from build123d import *

# Parameters (mm, degrees)
SKETCH1_R           = 1.5
BOSS_EXTRUDE1_DEPTH = 1.1
SKETCH2_R           = 2.455
BOSS_EXTRUDE2_DEPTH = 7.365
DOME1_FACE_RADIUS   = 2.455
DOME1_HEIGHT        = 2.455
SKETCH9_W           = 6
SKETCH9_H           = 9.85
BOSS_EXTRUDE3_DEPTH = 5.52
BOSS_EXTRUDE4_DEPTH = 9.85


with BuildPart() as part:
    # Sketch1 → Boss-Extrude1 (new body)
    with BuildSketch(Plane(origin=(0, 0, 0), x_dir=(1, 0, 0), z_dir=(0, 1, 0))):
        with BuildLine():
            Line((3.5, 0), (26.5, 0))
            ThreePointArc((26.5, 0), (28.974873734, 1.025126266), (30, 3.5))
            Line((30, 3.5), (30, 18.5))
            ThreePointArc((30, 18.5), (28.974873734, 20.974873734), (26.5, 22))
            Line((26.5, 22), (3.5, 22))
            ThreePointArc((3.5, 22), (1.025126266, 20.974873734), (0, 18.5))
            Line((0, 18.5), (0, 3.5))
            ThreePointArc((0, 3.5), (1.025126266, 1.025126266), (3.5, 0))
        make_face()
        with Locations(Location((26.5, 18.5, 0), (0, 0, 270))):
            Circle(SKETCH1_R, mode=Mode.SUBTRACT)
        with Locations(Location((26.5, 3.5, 0), (0, 0, 270))):
            Circle(SKETCH1_R, mode=Mode.SUBTRACT)
    extrude(amount=BOSS_EXTRUDE1_DEPTH)

    # Sketch2 → Boss-Extrude2 (add)
    with BuildSketch(Plane(origin=(0, 1.1, 0), x_dir=(1, 0, 0), z_dir=(0, 1, 0))):
        with Locations(Location((17.375, 11, 0), (0, 0, 270))):
            Circle(SKETCH2_R)
    extrude(amount=BOSS_EXTRUDE2_DEPTH)

    # Dome1: a dome of height H over a round flat face of radius A is a cap of a sphere of radius (A * A + H * H) / (2 * H)
    dome1_r = (DOME1_FACE_RADIUS * DOME1_FACE_RADIUS + DOME1_HEIGHT * DOME1_HEIGHT) / (2 * DOME1_HEIGHT)
    dome1_base = Plane((17.375, 8.465, -11), z_dir=(0, 1, 0))
    with Locations(dome1_base.offset(DOME1_HEIGHT - dome1_r)):
        dome1_ball = Sphere(dome1_r, mode=Mode.PRIVATE)
    add(split(dome1_ball, bisect_by=dome1_base, keep=Keep.TOP, mode=Mode.PRIVATE))

    # Sketch9 → Boss-Extrude3 (add)
    with BuildSketch(Plane(origin=(0, 1.1, 0), x_dir=(1, 0, 0), z_dir=(0, 1, 0))):
        with Locations((3, 11)):
            Rectangle(SKETCH9_W, SKETCH9_H)
    extrude(amount=BOSS_EXTRUDE3_DEPTH)

    # Sketch11 → Boss-Extrude4 (add)
    with BuildSketch(Plane(origin=(0, 0, -15.925), x_dir=(-1, 0, 0), z_dir=(0, 0, -1))):
        Polygon((0, 1.1), (-7.61, 1.1), (-6, 6.62), (0, 6.62), align=None)
    extrude(amount=-BOSS_EXTRUDE4_DEPTH)


solid = part.part
The listing builds one solid part. Answer for the finished solid, in the listing's coordinates (mm). A direction names the side the tool comes from. Give positions to 0.01 mm unless a question says otherwise; leave off trailing zeros. Loops run counter-clockwise (first coordinate to the right, second up) from the corner with the lowest first, then second, coordinate; pieces in that order, holes last. Notation, with made-up numbers: (85, -6) - (113, -6) arc R20 cw to (113, 18) - close; hole circle Ø10 at (23.5, 42.25). An arc over 180 degrees is marked (long way). Answer as a JSON object with one key per item and string values.
1. A cutting plane is placed at A-A (z = -11). Write down the section's boundary in (x, y) (3 decimals).
Determined:
{"outline": "(0, 0) - (30, 0) - (30, 1.1) - (19.83, 1.1) - (19.83, 8.465) arc R2.455 ccw to (14.92, 8.465) - (14.92, 1.1) - (7.61, 1.1) - (6, 6.62) - (0, 6.62) - close"}
2. Flat-ended cylindrical pins translate along their axes: pin 1 Ø1.7 at (x, y) = (3.5, 5) entering from -Z (3 decimals); pin 2 Ø1.7 at (x, y) = (3.5, 3) entering from +Z (3 decimals); pin 3 Ø6.5 at (x, z) = (2, -10.5) entering from +Y. Find the tip coordinate at first contact, or state that the pin passes through.
Determined:
{"pin 1": "z = -15.925", "pin 2": "z = -6.075", "pin 3": "y = 6.62"}
3. A cutting plane is placed at D-D (x = 9.5). Write down the section's boundary in (y, z), then the cut area to 3 significant figures.
Determined:
{"outline": "(0, -22) - (1.1, -22) - (1.1, 0) - (0, 0) - close", "area": "24.2 mm²"}
4. For a pull along X with two mould halves and no side action, classify faces 5 (the cylindrical face through (29, 0.54, -20.95)), 6 (the cylindrical face through (27.765, 0.542, -2.694)), 7 (the cylindrical face through (1, 0.54, -1.05)), 8 (the flat face through (4, 4, -15.925)) as pulls with the +X half, pulls with the -X half, needs draft (parallel to the pull), parting line crosses it, or undercut.
Determined:
{"face 5": "pulls with the +X half", "face 6": "undercut", "face 7": "pulls with the -X half", "face 8": "needs draft"}
5. A cutting plane is placed at C-C (y = 8). Write down the section's boundary in (x, z) (3 decimals).
Determined:
{"outline": "circle Ø4.91 at (17.375, -11)"}
6. Find the intervals of material crossed by L1, parallel to X at y = 0.75, z = -18.5; L2, parallel to Y at x = 8.5, z = -13; L3, parallel to Z at x = 6.75, y = 2 (3 decimals), in increasing order. Write a range as [from, to].
Determined:
{"L1": "[0, 25], [28, 30]", "L2": "[0, 1.1]", "L3": "[-15.925, -6.075]"}
7. A cutting plane is placed at B-B (x = 18.5). Write down the section's boundary in (y, z) (3 decimals), then the cut area to 3 significant figures.
Determined:
{"outline": "(0, -22) - (1.1, -22) - (1.1, -13.182) - (8.465, -13.182) arc R2.182 ccw to (8.465, -8.818) - (1.1, -8.818) - (1.1, 0) - (0, 0) - close", "area": "63.8 mm²"}
8. For faces 1 (the flat face through (6.816, 3.821, -11.069)), 2 (the flat face through (3, 6.62, -11)), 3 (the cylindrical face through (18.112, 4.731, -8.658)), 4 (the flat face through (4, 4, -6.075)), determine the directions among +Z, -Z, +X, -X, +Y, -Y from which every point of the face is accessible in a straight line to the end or side of a thin tool.
Determined:
{"face 1": "+Z, -Z, +Y", "face 2": "+Z, -Z, -X, +Y", "face 3": "+Y", "face 4": "+Z, +X, -X, +Y"}
